Model file for the job. Use its own axes, mm. A direction names the side the tool comes from. Round coordinates to 2 decimals unless told otherwise and drop trailing zeros. Write each loop counter-clockwise with the first axis right and the second up, starting at its lowest first coordinate (ties: lowest second). Pieces come first, ordered by that corner, then holes.
```python
from build123d import *

# Parameters (mm, degrees)
SKETCH1_W           = 7.8
SKETCH1_H           = 3.9
BOSS_EXTRUDE1_DEPTH = 20
CUT_EXTRUDE1_DEPTH  = 15
SKETCH4_W           = 6
SKETCH4_H           = 1
CUT_EXTRUDE2_DEPTH  = 2
SKETCH6_W           = 1.9
SKETCH6_H           = 1.9
BOSS_EXTRUDE3_DEPTH = 2
SKETCH7_W           = 2
SKETCH7_H           = 2
CUT_EXTRUDE3_DEPTH  = 2


with BuildPart() as part:
    # Sketch1 → Boss-Extrude1 (new body)
    with BuildSketch(Plane(origin=(0, 0, 0), x_dir=(1, 0, 0), z_dir=(0, 1, 0))):
        with Locations((1.261259263, 0.247513191)):
            Rectangle(SKETCH1_W, SKETCH1_H)
    extrude(amount=BOSS_EXTRUDE1_DEPTH)

    # Sketch3 → Cut-Extrude1 (cut)
    with BuildSketch(Plane.XZ):
        with BuildLine():
            Line((-0.238740737, -2.197513191), (2.761259263, -2.197513191))
            ThreePointArc((2.761259263, -2.197513191), (2.710148003, -1.809284623), (2.560297369, -1.447513191))
            Line((2.560297369, -1.447513191), (-0.037778842, -1.447513191))
            ThreePointArc((-0.037778842, -1.447513191), (-0.187629476, -1.809284623), (-0.238740737, -2.197513191))
        make_face()
        with BuildLine():
            Line((2.761259263, -2.197513191), (4.261259263, -2.197513191))
            Line((4.261259263, -2.197513191), (4.261259263, -1.447513191))
            Line((4.261259263, -1.447513191), (2.560297369, -1.447513191))
            ThreePointArc((2.560297369, -1.447513191), (2.710148003, -1.809284623), (2.761259263, -2.197513191))
        make_face()
        with BuildLine():
            Line((-0.037778842, -1.447513191), (2.560297369, -1.447513191))
            ThreePointArc((2.560297369, -1.447513191), (1.261259263, -0.697513191), (-0.037778842, -1.447513191))
        make_face()
        with BuildLine():
            Line((-1.738740737, -2.197513191), (-0.238740737, -2.197513191))
            ThreePointArc((-0.238740737, -2.197513191), (-0.187629476, -1.809284623), (-0.037778842, -1.447513191))
            Line((-0.037778842, -1.447513191), (-1.738740737, -1.447513191))
            Line((-1.738740737, -1.447513191), (-1.738740737, -2.197513191))
        make_face()
    extrude(amount=-CUT_EXTRUDE1_DEPTH, mode=Mode.SUBTRACT)

    # Sketch4 → Cut-Extrude2 (cut)
    with BuildSketch(Plane(origin=(0, 20, 0), x_dir=(1, 0, 0), z_dir=(0, 1, 0))):
        with Locations((1.261259263, 1.697513191)):
            Rectangle(SKETCH4_W, SKETCH4_H)
    extrude(amount=-CUT_EXTRUDE2_DEPTH, mode=Mode.SUBTRACT)

    # Sketch6 → Boss-Extrude3 (add)
    with BuildSketch(Plane(origin=(0, 0, -2.197513191), x_dir=(-1, 0, 0), z_dir=(0, 0, -1))):
        with Locations((-2.261259263, 16.5)):
            Rectangle(SKETCH6_W, SKETCH6_H)
    extrude(amount=BOSS_EXTRUDE3_DEPTH)

    # Sketch7 → Cut-Extrude3 (cut)
    with BuildSketch(Plane(origin=(0, 0, -2.197513191), x_dir=(-1, 0, 0), z_dir=(0, 0, -1))):
        with Locations((-0.261259263, 16.5)):
            Rectangle(SKETCH7_W, SKETCH7_H)
    extrude(amount=-CUT_EXTRUDE3_DEPTH, mode=Mode.SUBTRACT)


solid = part.part
```
1) Pull direction X, two halves, no side cores. Call faces 4 (the face through (5.161, 10, 0)), 5 (the face through (-1.739, 19, -2)), 6 (the face through (1.311, 16, -3)), 7 (the face through (0, 15.5, -1)): released by +X, released by -X, zero draft, split by the parting line, or undercut.
2) Cut at C-C on y = 16.25. List the corners of the cut face in (x, z).
3) Cut at D-D on x = 0.5. List the corners of the cut face in (y, z), and give its area (3 significant figures).
4) Wall check: probe 1 along Z at (x, y) = (2.75, 15.5); probe 2 along Y at (x, z) = (1.5, -1); probe 3 along Y at (x, z) = (-0.5, -1). Give the ranges that are in metal, low to high.
5) Cut at A-A on y = 11.25. List the corners of the cut face in (x, z), and give its area (3 significant figures).
6) Which spindle directions (+Z, -Z, +X, -X, +Y, -Y) get a long thin tool onto all of the face, cutting with end or side? Do faces 1 (the face through (-1, 7, -1.448)), 2 (the face through (0, 17, -0.198)), 3 (the face through (2, 17.45, -3)). Say none if no direction does.
7) Cut at B-B on x = 4. List the corners of the cut face in (y, z), and give its area (4 significant figures).
8) Flat gauge pins, fed straight in: pin 1 Ø2 at (x, z) = (2.5, -3.5) entering from -Y; pin 2 Ø2 at (x, y) = (3.5, 14.5) entering from -Z; pin 3 Ø0.6 at (y, z) = (16, -3) entering from +X. Where does each tip first touch, or does it go through?
Result sheet:
1. face 4: released by +X
1. face 5: undercut
1. face 6: released by -X
1. face 7: undercut
2. outline: (-2.64, -2.2) - (-0.74, -2.2) - (-0.74, -0.2) - (1.26, -0.2) - (1.26, -2.2) - (1.31, -2.2) - (1.31, -4.2) - (3.21, -4.2) - (3.21, -2.2) - (5.16, -2.2) - (5.16, 1.7) - (-2.64, 1.7) - close
3. outline: (0, -0.91) - (15, -0.91) - (15, -2.2) - (15.5, -2.2) - (15.5, -0.2) - (17.5, -0.2) - (17.5, -2.2) - (18, -2.2) - (18, -1.2) - (20, -1.2) - (20, 1.7) - (0, 1.7) - close
3. area: 52.6 mm2
4. probe 1: z = -2.2 to 1.7
4. probe 2: y = 15 to 20
4. probe 3: y = 0 to 15.5, 17.5 to 20
5. outline: (-2.64, -2.2) - (-1.74, -2.2) - (-1.74, -1.45) - (-0.04, -1.45) arc R1.5 cw to (2.56, -1.45) - (4.26, -1.45) - (4.26, -2.2) - (5.16, -2.2) - (5.16, 1.7) - (-2.64, 1.7) - close
5. area: 24.5 mm2
6. face 1: -Z, -Y
6. face 2: -Z
6. face 3: -Z, +X, -X, +Y
7. outline: (0, -1.45) - (15, -1.45) - (15, -2.2) - (18, -2.2) - (18, -1.2) - (20, -1.2) - (20, 1.7) - (0, 1.7) - close
7. area: 64.75 mm2
8. pin 1: stops at y = 15.55
8. pin 2: stops at z = -2.2
8. pin 3: stops at x = 3.21
